Design review of the part built by this model. Coordinates are the model's own, in mm. Face numbers are marked on the shaded views. A direction names the side the tool comes from. Round coordinates to 2 decimals unless told otherwise and drop trailing zeros. Write each loop counter-clockwise with the first axis right and the second up, starting at its lowest first coordinate (ties: lowest second). Pieces come first, ordered by that corner, then holes. Notation, with made-up numbers: M 11.5,8 L 46.5,8 A23 ccw 46.5,43 Z; hole C -39,-10.5 d11. An arc over 180 degrees is marked long. Use CSV: the item, a comma, the result in double quotes.
from build123d import *

# Parameters (mm, degrees)
SKETCH1_R               = 6
BOSS_EXTRUDE1_DEPTH     = 20
SKETCH2_R               = 3.4
CUT_EXTRUDE1_DEPTH      = 13.55
SKETCH5_W               = 1.550685087
SKETCH5_H               = 7.184215806
BOSS_EXTRUDE2_DEPTH     = 13.55
SKETCH7_W               = 9.286501956
SKETCH7_H               = 19.909960041
BOSS_EXTRUDE3_DEPTH     = 10
SKETCH6_R               = 2
CUT_EXTRUDE2_DEPTH      = 1
CUT_EXTRUDE2_DEPTH_BACK = 13.55
CUT_EXTRUDE3_DEPTH      = 10
CUT_EXTRUDE3_DEPTH_BACK = 10


with BuildPart() as part:
    # Sketch1 → Boss-Extrude1 (new body)
    with BuildSketch(Plane(origin=(0, 0, 0), x_dir=(1, 0, 0), z_dir=(0, 1, 0))):
        Circle(SKETCH1_R)
    extrude(amount=BOSS_EXTRUDE1_DEPTH)

    # Sketch2 → Cut-Extrude1 (cut)
    with BuildSketch(Plane(origin=(0, 20, 0), x_dir=(1, 0, 0), z_dir=(0, 1, 0))):
        Circle(SKETCH2_R)
    extrude(amount=-CUT_EXTRUDE1_DEPTH, mode=Mode.SUBTRACT)

    # Sketch5 → Boss-Extrude2 (add)
    with BuildSketch(Plane(origin=(0, 18.26, 0), x_dir=(1, 0, 0), z_dir=(0, 1, 0))):
        with Locations((3.375342544, 0.020519704)):
            Rectangle(SKETCH5_W, SKETCH5_H)
    extrude(amount=-BOSS_EXTRUDE2_DEPTH)

    # Sketch7 → Boss-Extrude3 (add)
    with BuildSketch(Plane.ZY.offset(-2.6)):
        with Locations((-0.005218197, 9.954980021)):
            Rectangle(SKETCH7_W, SKETCH7_H)
    extrude(amount=-BOSS_EXTRUDE3_DEPTH)

    # Sketch6 → Cut-Extrude2 (cut, two sides)
    with BuildSketch(Plane.ZY.offset(-2.6)) as cut_extrude2_sk:
        with Locations((0, 10.236925537)):
            Circle(SKETCH6_R)
    extrude(amount=CUT_EXTRUDE2_DEPTH, mode=Mode.SUBTRACT)
    extrude(cut_extrude2_sk.sketch, amount=-CUT_EXTRUDE2_DEPTH_BACK, mode=Mode.SUBTRACT)

    # Sketch9 → Cut-Extrude3 (cut, two sides)
    with BuildSketch(Plane.XY) as cut_extrude3_sk:
        Polygon((11.063430227, 10.236925537), (11.063430227, 5.861925537), (4.943430227, 5.861925537), (4.943430227, 10.236925537), (4.943430227, 14.611925537), (11.063430227, 14.611925537), align=None)
    extrude(amount=CUT_EXTRUDE3_DEPTH, mode=Mode.SUBTRACT)
    extrude(cut_extrude3_sk.sketch, amount=-CUT_EXTRUDE3_DEPTH_BACK, mode=Mode.SUBTRACT)


solid = part.part
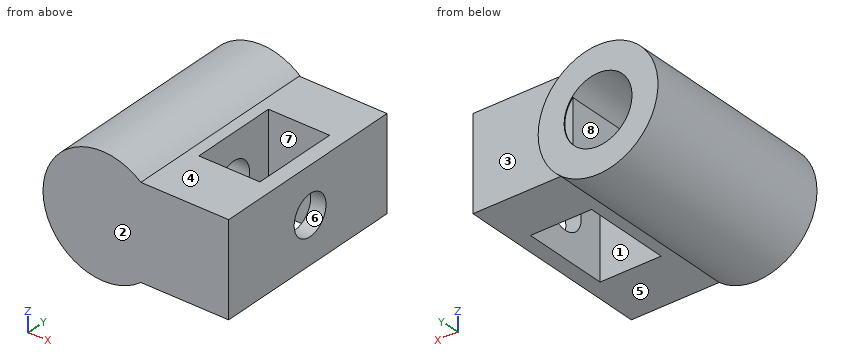
1) Add section D-D on y = 16.25. Write out the cut boundary in (x, z).
Answers:
outline,"M 3.79,-4.65 L 12.6,-4.65 L 12.6,4.64 L 3.81,4.64 A6 ccw long Z; hole M 2.6,-2.19 L 2.6,2.19 A3.4 ccw long Z"
2) Add section A-A on z = 0. Write out the cut boundary in (x, y), then the cut area to 3 significant figures.
Answers:
outline,"M -6,0 L 12.6,0 L 12.6,8.24 L 11.06,8.24 L 11.06,5.86 L 4.94,5.86 L 4.94,8.24 L 2.6,8.24 L 2.6,6.45 L -3.4,6.45 L -3.4,20 L -6,20 Z; M 2.6,12.24 L 4.94,12.24 L 4.94,14.61 L 11.06,14.61 L 11.06,12.24 L 12.6,12.24 L 12.6,19.91 L 6,19.91 L 6,20 L 3.4,20 L 3.4,19.91 L 2.6,19.91 Z"
area,"221 mm²"
3) Add section B-B on x = 6.5. Write out the cut boundary in (y, z).
Answers:
outline,"M 0,-4.65 L 5.86,-4.65 L 5.86,4.64 L 0,4.64 Z; M 14.61,-4.65 L 19.91,-4.65 L 19.91,4.64 L 14.61,4.64 Z"
4) For pin 1 Ø8 at (x, y) = (7, 17.5) entering from -Z; pin 2 Ø3 at (y, z) = (12, 3.5) entering from -X; pin 3 Ø4 at (x, y) = (4, 5.5) entering from -Z, all flat-tipped, find the tip position at first contact; note any pin that passes through.
Answers:
pin 1,"z = -5.2"
pin 2,"x = -5.66"
pin 3,"z = -5.66"
5) Machinability: for the marked faces 4, 5, 6, 7 and 8, which of the approach directions +Z, -Z, +X, -X, +Y, -Y give a long, thin tool a straight path to every point of the face, cutting with its end or side? Answer none if there is none.
Answers:
face 4,"+Z, +X, +Y, -Y"
face 5,"-Z, +X, +Y, -Y"
face 6,"+X"
face 7,"+Z, -Z"
face 8,"+Y"
6) The part is to be moulded in two halves that separate along Y. For the marked faces 1, 2 and 3, say which applies: released by +Y, released by -Y, zero draft, split by the parting line, or undercut.
Answers:
face 1,"undercut"
face 2,"released by -Y"
face 3,"released by +Y"
7) Wall thickness on line 1 along X through (y, z) = (14.25, 0); line 2 along Y through (x, z) = (7, 1); line 3 along Y through (x, z) = (4.3, 0): over which ranges is each line inside the solid? List them lowest first. Write a range as [from, to].
Answers:
line 1,"[-6, -3.4], [2.6, 4.94], [11.06, 12.6]"
line 2,"[0, 5.86], [14.61, 19.91]"
line 3,"[0, 8.24], [12.24, 20]"
8) Add section C-C on x = 0. Write out the cut boundary in (y, z), then the cut area to 3 significant figures.
Answers:
outline,"M 0,-6 L 20,-6 L 20,-3.4 L 6.45,-3.4 L 6.45,3.4 L 20,3.4 L 20,6 L 0,6 Z"
area,"148 mm²"
